```python
from build123d import *

# Parameters (mm, degrees)
BOSS_EXTRUDE1_DEPTH            = 17.4
CUT_EXTRUDE1_DEPTH             = 12.75
BOSS_EXTRUDE2_DEPTH            = 5
BOSS_EXTRUDE3_REACH            = 51.227
BOSS_EXTRUDE4_DEPTH            = 4.65
BOSS_EXTRUDE5_DEPTH            = 4.65
BOSS_EXTRUDE6_REACH            = 51.227
BOSS_EXTRUDE7_DEPTH            = 4.65
BOSS_EXTRUDE8_START            = -4.65
BOSS_EXTRUDE8_DEPTH            = 4.65
CHAMFER2_SIZE                  = 2
SKETCH10_R                     = 3.525
CUT_EXTRUDE2_DEPTH             = 50.226923528
CUT_EXTRUDE3_DEPTH             = 0.381
BOSS_EXTRUDE9_DEPTH            = 3
BOSS_EXTRUDE10_START           = -5
BOSS_EXTRUDE10_DEPTH           = 5
M3_CLEARANCE_HOLE1_D           = 3.6
M3_CLEARANCE_HOLE2_D           = 3.6
CHAMFER5_SIZE                  = 1
CUT_EXTRUDE4_REACH             = 52.009
CUT_EXTRUDE4_DIRECTION_2_REACH = 52.009
CHAMFER6_SIZE                  = 1


with BuildPart() as part:
    # Sketch1 → Boss-Extrude1 (new, symmetric)
    with BuildSketch(Plane(origin=(0, 0, 0), x_dir=(0, 0, -1), z_dir=(1, 0, 0))):
        with BuildLine():
            Line((0, 17.5), (-10, 17.5))
            ThreePointArc((-10, 17.5), (-20, 0), (-10, -17.5))
            Line((-10, -17.5), (0, -17.5))
            ThreePointArc((0, -17.5), (10, 0), (0, 17.5))
        make_face()
    extrude(amount=BOSS_EXTRUDE1_DEPTH, both=True)

    # Sketch2 → Cut-Extrude1 (cut, symmetric)
    with BuildSketch(Plane(origin=(0, 0, 0), x_dir=(0, 0, -1), z_dir=(1, 0, 0))):
        with BuildLine():
            Line((-6, -17.5), (0, -17.5))
            ThreePointArc((0, -17.5), (10, 0), (0, 17.5))
            Line((0, 17.5), (-6, 17.5))
            ThreePointArc((-6, 17.5), (-16, 0), (-6, -17.5))
        make_face()
    extrude(amount=CUT_EXTRUDE1_DEPTH, both=True, mode=Mode.SUBTRACT)

    # Sketch3 → Boss-Extrude2 (add, symmetric)
    with BuildSketch(Plane(origin=(0, 0, 0), x_dir=(0, 0, -1), z_dir=(1, 0, 0))):
        with BuildLine():
            Line((-9.5, -17.5), (-9.5, -24))
            ThreePointArc((-9.5, -24), (-5, -28.5), (-0.5, -24))
            Line((-0.5, -24), (-0.5, -17.5))
            Line((-0.5, -17.5), (-9.5, -17.5))
        make_face()
    extrude(amount=BOSS_EXTRUDE2_DEPTH, both=True)

    # Boss-Extrude3: up to this face of the body (flat: up to its plane)
    boss_extrude3_end = Plane(part.part.faces().sort_by_distance((-17.4, 0, 5))[0])
    # Sketch4 → Boss-Extrude3 (add, up to the picked face)
    with BuildSketch(Plane(origin=(17.4, 0, 0), x_dir=(0, 0, -1), z_dir=(1, 0, 0)), mode=Mode.PRIVATE) as boss_extrude3_sk1:
        with BuildLine():
            Line((-13.437411512, -9.876147912), (0.981589269, -18.200961894))
            Line((0.981589269, -18.200961894), (0.808939539, -18.5))
            Line((0.808939539, -18.5), (-8.303030303, -18.5))
            Line((-8.303030303, -18.5), (-10, -17.5))
            ThreePointArc((-10, -17.5), (-14.227290753, -14.184221555), (-17.437411512, -9.876147912))
            Line((-17.437411512, -9.876147912), (-13.437411512, -9.876147912))
        make_face()
    boss_extrude3_tool1 = split(extrude(boss_extrude3_sk1.sketch, amount=-BOSS_EXTRUDE3_REACH, mode=Mode.PRIVATE), bisect_by=boss_extrude3_end, keep=Keep.BOTH, mode=Mode.PRIVATE)
    add(boss_extrude3_tool1.solids().sort_by(Axis((17.4, -14.739023, 9.130288), (-1, 0, 0)))[0])

    # Sketch5 → Boss-Extrude4 (add)
    with BuildSketch(Plane(origin=(17.4, 0, 0), x_dir=(0, 0, -1), z_dir=(1, 0, 0))):
        Polygon((5.425994541, -12.841240042), (0.808939539, -18.5), (-1.191060461, -18.5), (-1.191060461, -17.5), align=None)
    extrude(amount=-BOSS_EXTRUDE4_DEPTH)

    # Sketch6 → Boss-Extrude5 (add)
    with BuildSketch(Plane.ZY.offset(17.4)):
        Polygon((-5.425994541, -12.841240042), (-0.808939539, -18.5), (1.191060461, -18.5), (1.191060461, -17.5), align=None)
    extrude(amount=-BOSS_EXTRUDE5_DEPTH)

    # Boss-Extrude6: up to this face of the body (flat: up to its plane)
    boss_extrude6_end = Plane(part.part.faces().sort_by_distance((-17.4, -0.260518526, 4.968984896))[0])
    # Sketch7 → Boss-Extrude6 (add, up to the picked face)
    with BuildSketch(Plane(origin=(17.4, 0, 0), x_dir=(0, 0, -1), z_dir=(1, 0, 0)), mode=Mode.PRIVATE) as boss_extrude6_sk1:
        with BuildLine():
            Line((-10, 17.5), (-7.03030303, 19.25))
            Line((-7.03030303, 19.25), (16, 19.25))
            Line((16, 19.25), (16, 14.121852756))
            Line((16, 14.121852756), (3.105217997, 15.25))
            Line((3.105217997, 15.25), (-13.105217997, 15.25))
            ThreePointArc((-13.105217997, 15.25), (-11.605823563, 16.448441254), (-10, 17.5))
        make_face()
    boss_extrude6_tool1 = split(extrude(boss_extrude6_sk1.sketch, amount=-BOSS_EXTRUDE6_REACH, mode=Mode.PRIVATE), bisect_by=boss_extrude6_end, keep=Keep.BOTH, mode=Mode.PRIVATE)
    add(boss_extrude6_tool1.solids().sort_by(Axis((17.4, 17.022897, -3.374472), (-1, 0, 0)))[0])

    # Sketch8 → Boss-Extrude7 (add)
    with BuildSketch(Plane(origin=(17.4, 0, 0), x_dir=(0, 0, -1), z_dir=(1, 0, 0))):
        with BuildLine():
            Line((16, 14.121852756), (8.902736416, -6.585768423))
            ThreePointArc((8.902736416, -6.585768423), (9.319810717, 5.212488097), (3.105217997, 15.25))
            Line((3.105217997, 15.25), (16, 14.121852756))
        make_face()
    extrude(amount=-BOSS_EXTRUDE7_DEPTH)

    # Sketch9 → Boss-Extrude8 (add)
    with BuildSketch(Plane.ZY.offset(17.4).offset(BOSS_EXTRUDE8_START)):
        with BuildLine():
            Line((-16, 14.121852756), (-8.902736416, -6.585768423))
            ThreePointArc((-8.902736416, -6.585768423), (-9.319810717, 5.212488097), (-3.105217997, 15.25))
            Line((-3.105217997, 15.25), (-16, 14.121852756))
        make_face()
    extrude(amount=BOSS_EXTRUDE8_DEPTH)

    # Chamfer2
    chamfer2_edges = [part.edges().sort_by_distance(p)[0] for p in [
        (0, 19.25, -16),
    ]]
    chamfer(chamfer2_edges, length=CHAMFER2_SIZE)

    # Sketch10 → Cut-Extrude2 (cut, through all)
    with BuildSketch(Plane(origin=(17.4, 0, 0), x_dir=(0, 0, -1), z_dir=(1, 0, 0))):
        Circle(SKETCH10_R)
    extrude(amount=-CUT_EXTRUDE2_DEPTH, mode=Mode.SUBTRACT)

    # Sketch11 → Cut-Extrude3 (cut, symmetric)
    with BuildSketch(Plane(origin=(0, 0, 0), x_dir=(0, 0, -1), z_dir=(1, 0, 0))):
        with BuildLine():
            Line((-9.5, -17.5), (-9.5, -24))
            ThreePointArc((-9.5, -24), (-5, -28.5), (-0.5, -24))
            Line((-0.5, -24), (-0.5, -17.5))
            Line((-0.5, -17.5), (-9.5, -17.5))
        make_face()
    extrude(amount=CUT_EXTRUDE3_DEPTH, both=True, mode=Mode.SUBTRACT)

    # Sketch12 → Boss-Extrude9 (add)
    with BuildSketch(Plane.XZ.offset(18.5)):
        with BuildLine():
            Line((-17.4, -0.808939539), (-21.4, -0.808939539))
            ThreePointArc((-21.4, -0.808939539), (-24.228427125, 0.362633337), (-25.4, 3.191060461))
            Line((-25.4, 3.191060461), (-25.4, 22.303030303))
            ThreePointArc((-25.4, 22.303030303), (0, 32.303030303), (25.4, 22.303030303))
            Line((25.4, 22.303030303), (25.4, 3.191060461))
            ThreePointArc((25.4, 3.191060461), (24.228427125, 0.362633337), (21.4, -0.808939539))
            Line((21.4, -0.808939539), (17.4, -0.808939539))
            Line((17.4, -0.808939539), (17.4, 8.303030303))
            Line((17.4, 8.303030303), (-17.4, 8.303030303))
            Line((-17.4, 8.303030303), (-17.4, -0.808939539))
        make_face()
    extrude(amount=-BOSS_EXTRUDE9_DEPTH)

    # Sketch13 → Boss-Extrude10 (add)
    with BuildSketch(Plane.ZY.offset(17.4).offset(BOSS_EXTRUDE10_START)):
        with BuildLine():
            Line((20, -15.5), (20, 0))
            ThreePointArc((20, 0), (18.116589611, -8.542032098), (12.815624628, -15.5))
            Line((12.815624628, -15.5), (12.815624628, -23.5))
            Line((12.815624628, -23.5), (20, -23.5))
            Line((20, -23.5), (20, -15.5))
        make_face()
    boss_extrude10 = extrude(amount=BOSS_EXTRUDE10_DEPTH)

    # Mirror1: Boss-Extrude10 across plane
    add(boss_extrude10.mirror(Plane(origin=(0, 0, 0), x_dir=(0, 0, 1), z_dir=(1, 0, 0))))

    # M3 Clearance Hole1 (through all)
    with Locations(Plane(origin=(0, -15.5, 0), x_dir=(1, 0, 0), z_dir=(0, 1, 0))):
        with Locations((0, -27.303030303), (-21.4, -9.191060461), (21.4, -9.191060461)):
            Hole(M3_CLEARANCE_HOLE1_D / 2)

    # M3 Clearance Hole2 (through all)
    with Locations(Plane(origin=(5, 0, 0), x_dir=(0, 0, -1), z_dir=(1, 0, 0))):
        with Locations((-5, -24)):
            Hole(M3_CLEARANCE_HOLE2_D / 2)

    # Chamfer5
    chamfer5_edges = [part.edges().sort_by_distance(p)[0] for p in [
        (12.75, 0, 3.525),
        (-12.75, 0, 3.525),
        (-17.4, 0, 3.525),
        (17.4, 0, 3.525),
    ]]
    chamfer(chamfer5_edges, length=CHAMFER5_SIZE)

    # Cut-Extrude4: up to this face of the body (flat: up to its plane)
    cut_extrude4_end = Plane(part.part.faces().sort_by_distance((-12.75, 0, 4.990087357))[0])
    # Sketch18 → Cut-Extrude4 (cut, up to the picked face)
    with BuildSketch(Plane(origin=(0, 0, 0), x_dir=(0, 0, -1), z_dir=(1, 0, 0)), mode=Mode.PRIVATE) as cut_extrude4_sk1:
        with BuildLine():
            Line((-0.5, -18.5), (1.499538462, -18.5))
            Line((1.499538462, -18.5), (-0.232112642, -17.500230769))
            ThreePointArc((-0.232112642, -17.500230769), (0.017518635, -18.102893984), (-0.5, -18.5))
        make_face()
    cut_extrude4_tool1 = split(extrude(cut_extrude4_sk1.sketch, amount=-CUT_EXTRUDE4_REACH, mode=Mode.PRIVATE), bisect_by=cut_extrude4_end, keep=Keep.BOTH, mode=Mode.PRIVATE)
    add(cut_extrude4_tool1.solids().sort_by(Axis((0, -18.22087, -0.457813), (-1, 0, 0)))[0], mode=Mode.SUBTRACT)

    # Cut-Extrude4 direction 2: up to this face of the body (flat: up to its plane)
    cut_extrude4_direction_2_end = Plane(part.part.faces().sort_by_distance((12.75, 0, 4.990087357))[0])
    # Sketch18 → Cut-Extrude4 direction 2 (cut, up to the picked face)
    with BuildSketch(Plane(origin=(0, 0, 0), x_dir=(0, 0, -1), z_dir=(1, 0, 0)), mode=Mode.PRIVATE) as cut_extrude4_direction_2_sk1:
        with BuildLine():
            Line((-0.5, -18.5), (1.499538462, -18.5))
            Line((1.499538462, -18.5), (-0.232112642, -17.500230769))
            ThreePointArc((-0.232112642, -17.500230769), (0.017518635, -18.102893984), (-0.5, -18.5))
        make_face()
    cut_extrude4_direction_2_tool1 = split(extrude(cut_extrude4_direction_2_sk1.sketch, amount=CUT_EXTRUDE4_DIRECTION_2_REACH, mode=Mode.PRIVATE), bisect_by=cut_extrude4_direction_2_end, keep=Keep.BOTH, mode=Mode.PRIVATE)
    add(cut_extrude4_direction_2_tool1.solids().sort_by(Axis((0, -18.22087, -0.457813), (1, 0, 0)))[0], mode=Mode.SUBTRACT)

    # Chamfer6
    chamfer6_edges = [part.edges().sort_by_distance(p)[0] for p in [
        (-17.4, -23.5, 16.407812314),
        (-12.4, -23.5, 16.407812314),
        (-14.9, -23.5, 20),
        (-14.9, -23.5, 12.815624628),
        (14.9, -23.5, 20),
        (12.4, -23.5, 16.407812314),
        (17.4, -23.5, 16.407812314),
        (14.9, -23.5, 12.815624628),
    ]]
    chamfer(chamfer6_edges, length=CHAMFER6_SIZE)


solid = part.part
```
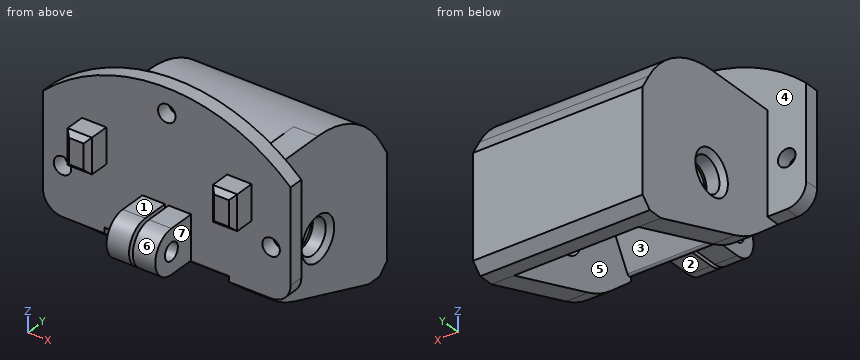
Geometry: final body of the model. Coordinates: model frame, mm. Face numbers are marked on the shaded views. A direction names the side the tool comes from. Give positions to 0.01 mm unless a question says otherwise; leave off trailing zeros. Loops run counter-clockwise (first coordinate to the right, second up) from the corner with the lowest first, then second, coordinate; pieces in that order, holes last. Notation, with made-up numbers: (-32.5, 76.5) -> (18.5, 76.5) arc R23 ccw to (18.5, 111.5) -> close; hole circle Ø3 at (-34.5, 78.25). An arc over 180 degrees is marked (long way). Use one line per item in the form item = value.
Item 1: Section query A-A on y = -21.5. Output: boundary loops of the cut face in (x, z), and give its area (3 significant figures).
A:
outline = (-17.4, 12.82) -> (-12.4, 12.82) -> (-12.4, 20) -> (-17.4, 20) -> close; (-5, 0.5) -> (-0.38, 0.5) -> (-0.38, 9.5) -> (-5, 9.5) -> close; (0.38, 0.5) -> (5, 0.5) -> (5, 9.5) -> (0.38, 9.5) -> close; (12.4, 12.82) -> (17.4, 12.82) -> (17.4, 20) -> (12.4, 20) -> close
area = 155 mm^2
Item 2: Section query D-D on y = 1. Give the number of separate pieces and of enclosed holes in the cut face, and give its area (3 significant figures).
A:
separate_pieces = 3
enclosed_holes = 0
area = 328 mm^2
Item 3: Pin query (flat end, axial travel): P1, Ø3, axis at x = 16, z = 22.5, coming from the -Y side; P2, Ø5.5, axis at x = 14, y = -8, coming from the +Z side; P3, Ø5, axis at x = 2, y = -21.5, coming from the -Z side. Return the tip coordinate at first contact, or that it passes through.
A:
P1 = -18.5
P2 = 20
P3 = 0.5
Item 4: Draft query along Y for the marked faces 5, 6 and 7. Return one class per face: pulls with the +Y half, pulls with the -Y half, needs draft (parallel to the pull), parting line crosses it, or undercut.
A:
face_5 = undercut
face_6 = pulls with the -Y half
face_7 = needs draft
Item 5: Access query for the marked faces 1, 2, 3 and 4. Directions: +Z, -Z, +X, -X, +Y, -Y. A direction counts if a zero-diameter tool reaches every point of the face in a straight line with its end or side. Return the directions, or none.
A:
face_1 = +Z, +X, -X, -Y
face_2 = -Z, +X, -X, -Y
face_3 = -Z
face_4 = +Z
Item 6: Line query: probe 1 along X at (y, z) = (5, -12.5); probe 2 along Y at (x, z) = (1.95, 5). Output: solid intervals per line, ascending.
A:
probe_1 = -17.4 to -12.75, 12.75 to 17.4
probe_2 = -28.5 to -25.8, -22.2 to -14.75, 15.25 to 19.25
Item 7: Section query C-C on z = -6.5. Output: boundary loops of the cut face in (x, y), and give its area (3 significant figures).
A:
outline = (-17.4, -11.4) -> (-12.75, -11.4) -> (-12.75, 14.95) -> (12.75, 14.95) -> (12.75, -11.4) -> (17.4, -11.4) -> (17.4, 19.25) -> (-17.4, 19.25) -> close
area = 395 mm^2
